Could you check a few things on this model? Use its own coordinates, in mm. A direction names the side the tool comes from. Give positions to 0.01 mm unless a question says otherwise; leave off trailing zeros. Order: outer loops, then holes, each group sorted by start corner. A loop starts at its lowest first (then second) coordinate and runs counter-clockwise, first axis right, second up. Notation, with made-up numbers: M -23,-10 L 18,-10 A10 ccw 18,2 Z; hole C 61.5,65.5 d5. An arc over 180 degrees is marked long. Use a Markdown table: item, result. Add a question column.
Item 1: If we mould it in two halves opening along Z, with no side actions, what happens to faces 4 (the face through (-1.305, 2.521, 0.74)), 5 (the face through (0, -10, 0)), 6 (the face through (-3.233, 1.976, 1.341))? For each: released by +Z, released by -Z, zero draft, split by the parting line, or undercut.
Item 2: Suppose I cut it at C-C on y = -1.5. Write out the boundary of the cut face in (x, z), plus the area to 3 significant figures.
Item 3: If I drill on L1, parallel to Y at x = -0.5, z = -0.25; L2, parallel to Y at x = 0.5, z = 2.5; L3, parallel to X at y = 2.25, z = 1.25, over which ranges is the centre line in solid material (lowest first)? Write a range as from..to.
Item 4: I'm going to push flat-ended pins straight in: pin 1 Ø0.9 at (x, z) = (-0.5, -0.5) entering from +Y; pin 2 Ø1 at (x, y) = (-1.5, -2) entering from +Z; pin 3 Ø3 at (y, z) = (-2.5, -2) entering from -X. Where does each tip first touch, or does it pass through?
Item 5: Suppose I cut it at B-B on x = 0. Write out the boundary of the cut face in (y, z).
Item 6: Suppose I cut it at A-A on y = 3. Write out the boundary of the cut face in (x, z).
Item 7: For faces 1 (the face through (-1.5, 4, -0.8)), 2 (the face through (1.293, 2.521, 0.76)), 3 (the face through (0, -5, 2)), which set-ups out of +Z, -Z, +X, -X, +Y, -Y let a thin tool reach every point of the face, with its end or its side?
from build123d import *

# Parameters (mm, degrees)
CUT_EXTRUDE1_DEPTH = 3
CHAMFER1_SIZE      = 0.25


with BuildPart() as part:
    # Sketch1 → Revolve1 (revolve)
    with BuildSketch(Plane.XY):
        Polygon((0, 4), (-3.5, 4), (-3.5, 0), (-2, 0), (-2, -10), (0, -10), (0, 0), align=None)
    revolve(axis=Axis((0, -10, 0), (0, -1, 0)))

    # Sketch2 → Cut-Extrude1 (cut)
    with BuildSketch(Plane(origin=(0, 4, 0), x_dir=(1, 0, 0), z_dir=(0, 1, 0))):
        Polygon((0.866025404, 1.5), (-0.866025404, 1.5), (-1.732050808, 0), (-0.866025404, -1.5), (0.866025404, -1.5), (1.732050808, 0), align=None)
    extrude(amount=-CUT_EXTRUDE1_DEPTH, mode=Mode.SUBTRACT)

    # Chamfer1
    chamfer1_edges = [part.edges().sort_by_distance(p)[0] for p in [
        (2, -10, 0),
        (3.5, 0, 0),
        (3.5, 4, 0),
    ]]
    chamfer(chamfer1_edges, length=CHAMFER1_SIZE)


solid = part.part
Findings below:
| question | item | result |
|---|---|---|
| 1 | face 4 | undercut |
| 1 | face 5 | zero draft |
| 1 | face 6 | split by the parting line |
| 2 | outline | C 0,0 d4 |
| 2 | area | 12.6 mm^2 |
| 3 | L1 | y = -10..1 |
| 3 | L2 | y = 0..4 |
| 3 | L3 | x = -3.27..-1.01, 1.01..3.27 |
| 4 | pin 1 | stops at y = 1 |
| 4 | pin 2 | stops at z = 1.73 |
| 4 | pin 3 | stops at x = -1.94 |
| 5 | outline | M -10,-1.75 L -9.75,-2 L 0,-2 L 0,-3.25 L 0.25,-3.5 L 3.75,-3.5 L 4,-3.25 L 4,-1.5 L 1,-1.5 L 1,1.5 L 4,1.5 L 4,3.25 L 3.75,3.5 L 0.25,3.5 L 0,3.25 L 0,2 L -9.75,2 L -10,1.75 Z |
| 6 | outline | C 0,0 d7; hole M -1.73,0 L -0.87,-1.5 L 0.87,-1.5 L 1.73,0 L 0.87,1.5 L -0.87,1.5 Z |
| 7 | face 1 | +Z, -Z, +X, -X, +Y |
| 7 | face 2 | +Y |
| 7 | face 3 | -Y |
